from build123d import *

# Parameters (mm, degrees)
SKETCH1_R                = 35.5
SKETCH1_R_2              = 23.5
BOSS_EXTRUDE1_DEPTH      = 17
M6_CLEARANCE_HOLE1_D     = 6.6
M6_CLEARANCE_HOLE1_DEPTH = 17
CIRPATTERN1_COUNT        = 6


with BuildPart() as part:
    # Sketch1 → Boss-Extrude1 (new body)
    with BuildSketch(Plane(origin=(0, 0, 0), x_dir=(1, 0, 0), z_dir=(0, 1, 0))):
        Circle(SKETCH1_R)
        Circle(SKETCH1_R_2, mode=Mode.SUBTRACT)
    extrude(amount=BOSS_EXTRUDE1_DEPTH)

    # M6 Clearance Hole1
    with Locations(Plane(origin=(-29, 17, 0), x_dir=(0, 0, 1), z_dir=(0, 1, 0))):
        with Locations((0, 0)):
            m6_clearance_hole1 = Hole(M6_CLEARANCE_HOLE1_D / 2, depth=M6_CLEARANCE_HOLE1_DEPTH)

    # CirPattern1: M6 Clearance Hole1 ×6 about axis
    cirpattern1_axis = Axis((0, 0, 0), (0, 1, 0))
    for i in range(1, CIRPATTERN1_COUNT):
        add(m6_clearance_hole1.rotate(cirpattern1_axis, i * 360 / CIRPATTERN1_COUNT), mode=Mode.SUBTRACT)


solid = part.part
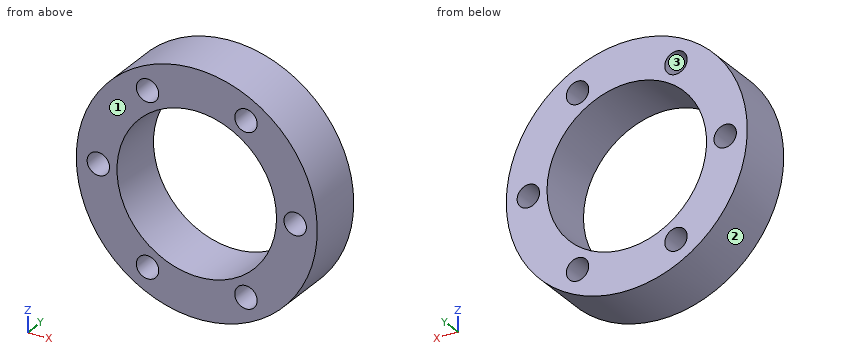
The listing builds one solid part. Answer for the finished solid, in the listing's coordinates (mm). Face numbers are marked on the shaded views. Give positions to 0.01 mm unless a question says otherwise; leave off trailing zeros. Loops run counter-clockwise (first coordinate to the right, second up) from the corner with the lowest first, then second, coordinate; pieces in that order, holes last.
Item 1: A cutting plane is placed at B-B (z = -17). Give the vertices of the cut face in (x, y), then the cut area to 3 significant figures.
Derived:
outline: (-31.16, 0) - (-16.22, 0) - (-16.22, 17) - (-31.16, 17) - close; (16.22, 0) - (31.16, 0) - (31.16, 17) - (16.22, 17) - close
area: 508 mm2
Item 2: Each of these flat-tipped pins is pushed along its axis until it touches: pin 1 Ø6 at (y, z) = (8, 25) entering from -X; pin 2 Ø4 at (y, z) = (2, -10.5) entering from +X; pin 3 Ø4 at (y, z) = (2.5, -12) entering from -X. Where does it stop, or does it pass through?
Derived:
pin 1: stops at x = -27.86
pin 2: stops at x = 34.47
pin 3: stops at x = -34.06
Item 3: A cutting plane is placed at C-C (y = 4.25). Give the vertices of the cut face in (x, z), then the cut area to 3 significant figures.
Derived:
outline: circle Ø71 at (0, 0); hole circle Ø6.6 at (-29, 0); hole circle Ø47 at (0, 0); hole circle Ø6.6 at (-14.5, -25.11); hole circle Ø6.6 at (-14.5, 25.11); hole circle Ø6.6 at (14.5, -25.11); hole circle Ø6.6 at (14.5, 25.11); hole circle Ø6.6 at (29, 0)
area: 2,020 mm2
Item 4: Determine the mould class of the marked faces 1, 2 and 3 for opening direction Z: +Z half, -Z half, draft (parallel to the pull), parting line (faces both ways), or undercut.
Derived:
face 1: draft
face 2: parting line
face 3: undercut
Item 5: Find the intervals of material crossed by line 1 along X through (y, z) = (12, 0); line 2 along X through (y, z) = (11.5, 24); line 3 along Z through (x, y) = (-14, 7.5), in increasing order.
Derived:
line 1: x = -35.5 to -32.3, -25.7 to -23.5, 23.5 to 25.7, 32.3 to 35.5
line 2: x = -26.16 to -17.61, -11.39 to 11.39, 17.61 to 26.16
line 3: z = -32.62 to -28.38, -21.85 to -18.87, 18.87 to 21.85, 28.38 to 32.62
Item 6: A cutting plane is placed at A-A (x = 0). Give the vertices of the cut face in (y, z), then the cut area to 3 significant figures.
Derived:
outline: (0, -35.5) - (17, -35.5) - (17, -23.5) - (0, -23.5) - close; (0, 23.5) - (17, 23.5) - (17, 35.5) - (0, 35.5) - close
area: 408 mm2
Item 7: A cutting plane is placed at D-D (x = 14.5). Give the vertices of the cut face in (y, z).
Derived:
outline: (0, -32.4) - (17, -32.4) - (17, -28.41) - (0, -28.41) - close; (0, -21.81) - (17, -21.81) - (17, -18.49) - (0, -18.49) - close; (0, 18.49) - (17, 18.49) - (17, 21.81) - (0, 21.81) - close; (0, 28.41) - (17, 28.41) - (17, 32.4) - (0, 32.4) - close
